Print and shaded views of the part. All mm, measured from the part's lowest x, y and z. Round coordinates to 2 decimals unless told otherwise and drop trailing zeros. Write each loop counter-clockwise with the first axis right and the second up, starting at its lowest first coordinate (ties: lowest second). Pieces come first, ordered by that corner, then holes. Notation, with made-up numbers: (-11, 37) -> (19, 37) arc R25 cw to (19, 66) -> close; hole circle Ø9 at (63.5, -30). An arc over 180 degrees is marked (long way). Use CSV: the item, a comma, the result in double quotes. Start each with the question number.
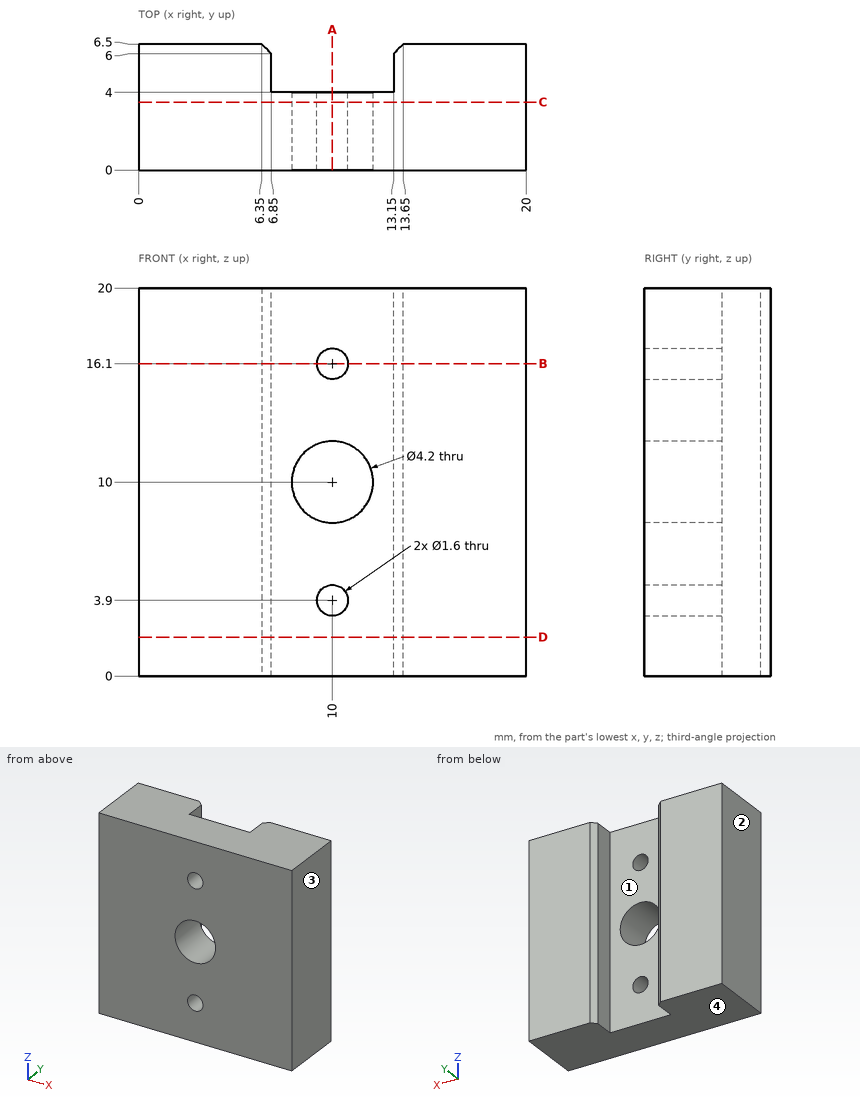
1. Band-saw the part on A-A (x = 10). List the corners of the cut face in (y, z).
2. Flat gauge pin, fed straight in: pin 1 (1.9 mm diameter, centred on x = 10, z = 6, fed in from +Y). Where does the tip first touch, or does it go through?
3. Band-saw the part on C-C (y = 3.5). List the corners of the cut face in (x, z).
4. Band-saw the part on D-D (z = 2). List the corners of the cut face in (x, y).
5. Band-saw the part on B-B (z = 16.1). List the corners of the cut face in (x, y).
6. Drill centre lines: line 1 along Z through (x, y) = (10, 1.35); line 2 along X through (y, z) = (5, 7.5); line 3 along Y through (x, z) = (10.75, 13.75). Where is each one in solid material? Low to high. Write a range as [from, to].
7. Pull direction X, two halves, no side cores. Call the marked faces 1, 2, 3 and 4: released by +X, released by -X, zero draft, split by the parting line, or undercut.
Answers below:
1,outline,"(0, 0) -> (4, 0) -> (4, 3.1) -> (0, 3.1) -> close; (0, 4.7) -> (4, 4.7) -> (4, 7.9) -> (0, 7.9) -> close; (0, 12.1) -> (4, 12.1) -> (4, 15.3) -> (0, 15.3) -> close; (0, 16.9) -> (4, 16.9) -> (4, 20) -> (0, 20) -> close"
2,pin 1,"stops at y = 4"
3,outline,"(0, 0) -> (20, 0) -> (20, 20) -> (0, 20) -> close; hole circle Ø4.2 at (10, 10); hole circle Ø1.6 at (10, 3.9); hole circle Ø1.6 at (10, 16.1)"
4,outline,"(0, 0) -> (20, 0) -> (20, 6.5) -> (13.65, 6.5) -> (13.15, 6) -> (13.15, 4) -> (6.85, 4) -> (6.85, 6) -> (6.35, 6.5) -> (0, 6.5) -> close"
5,outline,"(0, 0) -> (9.2, 0) -> (9.2, 4) -> (6.85, 4) -> (6.85, 6) -> (6.35, 6.5) -> (0, 6.5) -> close; (10.8, 0) -> (20, 0) -> (20, 6.5) -> (13.65, 6.5) -> (13.15, 6) -> (13.15, 4) -> (10.8, 4) -> close"
6,line 1,"z = [0, 3.1], [4.7, 7.9], [12.1, 15.3], [16.9, 20]"
6,line 2,"x = [0, 6.85], [13.15, 20]"
6,line 3,"y = [0, 4]"
7,face 1,"undercut"
7,face 2,"released by -X"
7,face 3,"released by +X"
7,face 4,"zero draft"
